CAD build for the part. Positions are in the model's coordinates, mm. A direction names the side the tool comes from. Round coordinates to 2 decimals unless told otherwise and drop trailing zeros. Write each loop counter-clockwise with the first axis right and the second up, starting at its lowest first coordinate (ties: lowest second). Pieces come first, ordered by that corner, then holes. Notation, with made-up numbers: (-32, 62) - (19, 62) arc R25 cw to (19, 89) - close; hole circle Ø2 at (11.5, 29.5). An arc over 180 degrees is marked (long way). Use one line per item in the form item = value. Start each with the question number.
Item 1: Tool access for faces 1 (the flat face through (10, -10, 0.6)), 2 (the flat face through (-7.2, 9.1, -1.5)), 3 (the flat face through (0, 0, -12.4)), 4 (the cylindrical face through (6.48, 13.21, 1.28)): list every direction of +Z, -Z, +X, -X, +Y, -Y with a clear straight run to the whole face (end or side of a thin tool).
Item 2: Band-saw the part on C-C, the plane z = 1. List the corners of the cut face in (x, y).
Item 3: Band-saw the part on B-B, the plane y = 0. List the corners of the cut face in (x, z), and give its area (3 significant figures).
Item 4: Band-saw the part on A-A, the plane x = 0. List the corners of the cut face in (y, z), and give its area (3 significant figures).
Item 5: Band-saw the part on D-D, the plane z = -6.5. List the corners of the cut face in (x, y) (1 decimal), and give its area (3 significant figures).
Item 6: Pin check, flat tips, straight feed: pin 1 (1.3 mm diameter, centred on y = 11.5, z = 1, fed in from -X); pin 2 (1 mm diameter, centred on x = 10.5, y = -3.5, fed in from +Z); pin 3 (7.5 mm diameter, centred on x = -4.5, y = -1, fed in from +Z). Stop position of each tip, or through.
Item 7: Drill centre lines: L1, parallel to X at y = 0, z = -0.25; L2, parallel to Z at x = -7, y = -1; L3, parallel to X at y = -3, z = -4.5. Where is each one in solid material? Low to high.
Item 8: Pull direction X, two halves, no side cores. Call faces 5 (the flat face through (-10, 10, 0.6)), 6 (the cylindrical face through (4.566, -14.498, -2.47)), 7 (the flat face through (5, -12, 2.6)): +X half, -X half, draft (parallel to the pull), parting line (faces both ways), or undercut.
from build123d import *

# Parameters (mm, degrees)
SKETCH002_W     = 12
SKETCH002_H     = 2.6
POCKET_DEPTH    = 7
POCKET001_DEPTH = 1.5
FILLET_R        = 1
CHAMFER_SIZE    = 0.75
CHAMFER001_SIZE = 1.4
SKETCH013_R     = 1
POCKET007_DEPTH = 2


with BuildPart() as part:
    # Sketch → Revolution (revolve)
    with BuildSketch(Plane.YZ):
        with BuildLine():
            Line((-12.2, 2.6), (-15.2, 2.6))
            Line((-15.2, 2.6), (-15.2, -7.4))
            ThreePointArc((-15.2, -7.4), (-13.735534, -10.935534), (-10.2, -12.4))
            Line((-10.2, -12.4), (0, -12.4))
            Line((0, -12.4), (0, -10.4))
            Line((0, -10.4), (-7.2, -10.4))
            ThreePointArc((-12.2, -5.4), (-10.735534, -8.935534), (-7.2, -10.4))
            Line((-12.2, -1.5), (-12.2, -5.4))
            Line((-10.7, -1.5), (-12.2, -1.5))
            Line((-10.7, 0), (-10.7, -1.5))
            Line((-10.7, 0), (-12.2, 0))
            Line((-12.2, 2.6), (-12.2, 0))
        make_face()
    revolve(axis=Axis((0, 0, 0), (0, 0, 1)))

    # Sketch002 (on DatumPlane) → Pocket (cut)
    with BuildSketch(Plane(origin=(0, 15.2, 0), x_dir=(-1, 0, 0), z_dir=(0, 1, 0))):
        with Locations((0, 1.3)):
            Rectangle(SKETCH002_W, SKETCH002_H)
    extrude(amount=-POCKET_DEPTH, mode=Mode.SUBTRACT)

    # Sketch003 → Pocket001 (cut)
    with BuildSketch(Plane.XY):
        with BuildLine():
            ThreePointArc((-4.172646, -11.46425), (6.1, -10.56551), (12.014655, -2.118508))
            Line((12.014655, -2.118508), (10.537443, -1.858036))
            ThreePointArc((-3.659616, -10.054711), (5.35, -9.266472), (10.537443, -1.858036))
            Line((-4.172646, -11.46425), (-3.659616, -10.054711))
        make_face()
    extrude(amount=-POCKET001_DEPTH, mode=Mode.SUBTRACT)

    # Fillet
    fillet_edges = [part.edges().sort_by_distance(p)[0] for p in [
        (6, 10.622617, 1.3),
        (6, 13.965672, 1.3),
        (-6, 10.622617, 1.3),
        (-6, 13.965672, 1.3),
    ]]
    fillet(fillet_edges, radius=FILLET_R)

    # Chamfer
    chamfer_edges = [part.edges().sort_by_distance(p)[0] for p in [
        (-5.35, 9.266472, -1.5),
    ]]
    chamfer(chamfer_edges, length=CHAMFER_SIZE)

    # Chamfer001
    chamfer001_edges = [part.edges().sort_by_distance(p)[0] for p in [
        (-3.659616, -10.054711, -0.375),
        (10.537443, -1.858036, -0.375),
    ]]
    chamfer(chamfer001_edges, length=CHAMFER001_SIZE)

    # Sketch013 → Pocket007 (cut)
    with BuildSketch(Plane.XY.offset(2.6)):
        with Locations((9.545942, 9.545942)):
            Circle(SKETCH013_R)
        with Locations((-9.545942, 9.545942)):
            Circle(SKETCH013_R)
        with Locations((-9.545942, -9.545942)):
            Circle(SKETCH013_R)
        with Locations((9.545942, -9.545942)):
            Circle(SKETCH013_R)
    extrude(amount=-POCKET007_DEPTH, mode=Mode.SUBTRACT)


solid = part.part
Determined:
q1.face_1 = +Z
q1.face_2 = none
q1.face_3 = -Z, +X, -X, +Y, -Y
q1.face_4 = +Z, +Y
q2.outline = (-7.49, 13.22) arc R15.2 ccw (long way) to (7.49, 13.22) arc R1 ccw to (6, 12.35) - (6, 11.19) arc R1 ccw to (6.47, 10.34) arc R12.2 cw (long way) to (-6.47, 10.34) arc R1 ccw to (-6, 11.19) - (-6, 12.35) arc R1 ccw to start; hole circle Ø2 at (-9.55, -9.55); hole circle Ø2 at (-9.55, 9.55); hole circle Ø2 at (9.55, -9.55); hole circle Ø2 at (9.55, 9.55)
q3.outline = (-15.2, -7.4) arc R5 ccw to (-10.2, -12.4) - (10.2, -12.4) arc R5 ccw to (15.2, -7.4) - (15.2, 2.6) - (12.2, 2.6) - (12.2, 0) - (10.7, 0) - (10.7, -0.75) - (11.45, -1.5) - (12.2, -1.5) - (12.2, -5.4) arc R5 cw to (7.2, -10.4) - (-7.2, -10.4) arc R5 cw to (-12.2, -5.4) - (-12.2, -1.5) - (-11.45, -1.5) - (-10.7, -0.75) - (-10.7, 0) - (-12.2, 0) - (-12.2, 2.6) - (-15.2, 2.6) - close
q3.area = 143 mm²
q4.outline = (-15.2, -7.4) arc R5 ccw to (-10.2, -12.4) - (10.2, -12.4) arc R5 ccw to (15.2, -7.4) - (15.2, 0) - (10.7, 0) - (10.7, -0.75) - (11.45, -1.5) - (12.2, -1.5) - (12.2, -5.4) arc R5 cw to (7.2, -10.4) - (-7.2, -10.4) arc R5 cw to (-12.2, -5.4) - (-12.2, 2.6) - (-15.2, 2.6) - close
q4.area = 133 mm²
q5.outline = circle Ø30.4 at (0, 0); hole circle Ø24.2 at (0, 0)
q5.area = 268 mm²
q6.pin_1 = -10.65
q6.pin_2 = -7.83
q6.pin_3 = -10.26
q7.L1 = -15.2 to -10.7, 10.7 to 15.2
q7.L2 = -12.4 to -10.4
q7.L3 = -14.9 to -11.83, 11.83 to 14.9
q8.face_5 = undercut
q8.face_6 = parting line
q8.face_7 = draft
